Design review of the part built by this model. Coordinates are the model's own, in mm. A direction names the side the tool comes from. Coordinates: 2 decimals unless noted, no trailing zeros. Write each loop counter-clockwise with the first axis right and the second up, starting at its lowest first coordinate (ties: lowest second). Pieces come first, ordered by that corner, then holes.
Q1. Clearance check with flat-ended pins moving along their axes: pin 1 Ø2.5 at (x, z) = (-13, 2) entering from -Y; pin 2 Ø6 at (y, z) = (-11, 1.5) entering from -X; pin 3 Ø3 at (x, z) = (-9.5, -3) entering from +Y; pin 4 Ø4 at (x, z) = (14.5, -0.5) entering from +Y. State where each tip first meets the part, or that it passes through.
Q2. Add section B-B, the plane z = 4.25. Give the boundary of the cut face in (x, y), plus the area to 3 significant figures.
Q3. Add section A-A, the plane x = 13.9. Give the boundary of the cut face in (y, z), plus the area to 3 significant figures.
Q4. Add section C-C, the plane y = -17.25. Give the boundary of the cut face in (x, z), plus the area to 3 significant figures.
Q5. Add section D-D, the plane x = 10. Give the boundary of the cut face in (y, z), plus the area to 3 significant figures.
Q6. Machinability: for faces 1 (the face through (15, -17, -0.65)), 2 (the face through (-12.6, -18, -0.1)), 3 (the face through (11.25, -8, 0)), 4 (the face through (-11.25, -8, 0)), which of the approach directions +Z, -Z, +X, -X, +Y, -Y give a long, thin tool a straight path to every point of the face, cutting with its end or side? Answer none if there is none.
Q7. To check wall thickness, follow probe 1 along Z at (x, y) = (-13.9, -16.7); probe 2 along X at (y, z) = (-16.5, 0); probe 3 along X at (y, z) = (-21.5, -1.5). State the ranges of each line that lie inside material, in increasing order.
Q8. The part is to be moulded in two halves that separate along X. For faces 5 (the face through (-12.9, -17, 0)), 6 (the face through (5, -28.7, 0)), 7 (the face through (2.91, -27.18, 0.1)), say which applies: +X half, -X half, draft (parallel to the pull), parting line (faces both ways), or undercut.
from build123d import *

# Parameters (mm, degrees)
F0_W          = 22.5
F0_H          = 11.8
F1_DEPTH      = 22.6
F2_W          = 2
F2_H          = 11.8
F3_DEPTH      = 5
F3_DEPTH_BACK = 27.5
F4_R          = 5.9
F5_DEPTH      = 3.1
F6_R          = 2.2332329477
F7_DEPTH      = 3
F9_D          = 2
F9_DEPTH      = 12
F9_TIP        = 0.600860619
F10_W         = 7.0652620957
F10_H         = 1.3
F10_W_2       = 9.383104834
F11_DEPTH     = 5


with BuildPart() as f1:
    # F0 (on Front) → F1 (new body)
    with BuildSketch(Plane.XZ):
        Rectangle(F0_W, F0_H)
    extrude(amount=F1_DEPTH)

    # F2 (on face) → F3 (join, two sides)
    with BuildSketch(Plane(origin=(-11.25, 0, 0), x_dir=(0, -1, 0), z_dir=(-1, 0, 0))) as f3_sk:
        with Locations((17, 0)):
            Rectangle(F2_W, F2_H)
    extrude(amount=F3_DEPTH)
    extrude(f3_sk.sketch, amount=-F3_DEPTH_BACK)

    # F4 (on face) → F5 (join)
    with BuildSketch(Plane.XZ.offset(22.6)):
        with Locations((5.1404135302, 0)):
            Circle(F4_R)
    extrude(amount=F5_DEPTH)

    # F6 (on face) → F7 (join)
    with BuildSketch(Plane.XZ.offset(25.7)):
        with Locations((5.1404135302, 0)):
            Circle(F6_R)
    extrude(amount=F7_DEPTH)

    # F9
    with Locations(Plane.XZ.offset(18)):
        with Locations((-13.9, 0), (13.9, 0)):
            Hole(F9_D / 2, depth=F9_DEPTH)
            with Locations((0, 0, -(F9_DEPTH + F9_TIP / 2))):  # 118° drill point
                Cone(0, F9_D / 2, F9_TIP, mode=Mode.SUBTRACT)

    # F10 (on face) → F11 (cut)
    with BuildSketch(Plane.XZ.offset(18)):
        with Locations((-19.7826310478, 0)):
            Rectangle(F10_W, F10_H)
        with BuildLine():
            ThreePointArc((-14.6599342077, -0.65), (-14.9, 0), (-14.6599342077, 0.65))
            Line((-14.6599342077, 0.65), (-16.25, 0.65))
            Line((-16.25, 0.65), (-16.25, -0.65))
            Line((-16.25, -0.65), (-14.6599342077, -0.65))
        make_face()
        with BuildLine():
            Line((-13.9321572616, -0.65), (-13.9321572616, 0.65))
            Line((-13.9321572616, 0.65), (-14.6599342077, 0.65))
            ThreePointArc((-14.6599342077, 0.65), (-14.9, 0), (-14.6599342077, -0.65))
            Line((-14.6599342077, -0.65), (-13.9321572616, -0.65))
        make_face()
        with Locations((18.763743341, 0)):
            Rectangle(F10_W_2, F10_H)
    extrude(amount=-F11_DEPTH, mode=Mode.SUBTRACT)


solid = f1.part
Here are the results:
1. pin 1: stops at y = -18
1. pin 2: stops at x = -11.25
1. pin 3: stops at y = 0
1. pin 4: stops at y = -16
2. outline: (-16.25, -18) - (-11.25, -18) - (-11.25, -22.6) - (1.05, -22.6) - (1.05, -25.7) - (9.23, -25.7) - (9.23, -22.6) - (11.25, -22.6) - (11.25, -18) - (16.25, -18) - (16.25, -16) - (11.25, -16) - (11.25, 0) - (-11.25, 0) - (-11.25, -16) - (-16.25, -16) - close
2. area: 554 mm2
3. outline: (-18, -5.9) - (-16, -5.9) - (-16, -1) - (-18, -1) - close; (-18, 1) - (-16, 1) - (-16, 5.9) - (-18, 5.9) - close
3. area: 19.6 mm2
4. outline: (-16.25, -5.9) - (16.25, -5.9) - (16.25, -0.65) - (14.66, -0.65) arc R1 cw (long way) to (14.66, 0.65) - (16.25, 0.65) - (16.25, 5.9) - (-16.25, 5.9) - (-16.25, 0.65) - (-14.66, 0.65) arc R1 cw (long way) to (-14.66, -0.65) - (-16.25, -0.65) - close
4. area: 374 mm2
5. outline: (-25.7, -3.35) - (-22.6, -3.35) - (-22.6, -5.9) - (0, -5.9) - (0, 5.9) - (-22.6, 5.9) - (-22.6, 3.35) - (-25.7, 3.35) - close
5. area: 287 mm2
6. face 1: +X, +Y, -Y
6. face 2: +Z, -Z, -X, -Y
6. face 3: +Z, -Z, +X, +Y
6. face 4: +Z, -Z, -X, +Y
7. probe 1: z = -5.9 to -1, 1 to 5.9
7. probe 2: x = -12.9 to 12.9
7. probe 3: x = -11.25 to 11.25
8. face 5: undercut
8. face 6: draft
8. face 7: parting line
